Autodesk Inventor part; units mm, degrees
ref_plane "YZ Plane" through (0, 0, 0) normal (1, 0, 0) x (0, 1, 0)
ref_plane "XZ Plane" through (0, 0, 0) normal (0, 1, 0) x (-1, 0, 0)
ref_plane "XY Plane" through (0, 0, 0) normal (0, 0, 1) x (1, 0, 0)
sketch "Schizzo1" plane through (0, 0, 0) normal (0, 0, 1) x (1, 0, 0)
  line L0 (0, 0) -> (90, 0)
  line L1 (90, 0) -> (90, -122)
  line L2 (90, -122) -> (0, -122)
  line L3 (0, -122) -> (0, 0)
  dimension "d0" = 90
  dimension "d1" = 122
extrude "Estrusione1" add sketch "Schizzo1" along normal blind 2.5
sketch "Schizzo2" plane through (0, 0, 2.5) normal (0, 0, 1) x (1, 0, 0)
  line L0 (90, 0) -> (0, 0)
  line L1 (0, -122) -> (90, -122)
  line L2 (90, 0) -> (87, 0)
  line L3 (87, -6.7) -> (12, -6.7)
  line L4 (12, -6.7) -> (12, -41.7)
  line L5 (12, -41.7) -> (87, -41.7)
  line L6 (87, -41.7) -> (87, -6.7)
  line L7 (0, -122) -> (10, -122)
  line L8 (10, -109) -> (83, -109)
  line L9 (83, -109) -> (83, -74)
  line L10 (83, -74) -> (10, -74)
  line L11 (10, -74) -> (10, -109)
  point P0 (87, -6.7)
  dimension "d6" = 75
  dimension "d7" = 35
  dimension "d10" = 73
  dimension "d11" = 35
extrude "Estrusione2" add sketch "Schizzo2" along normal blind 30
sketch "Schizzo3" plane through (0, 0, 2.5) normal (0, 0, 1) x (1, 0, 0)
  line L0 (90, -122) -> (90, 0)
  line L1 (90, 0) -> (0, 0)
  line L2 (90, 0) -> (90, -6)
  line L3 (90, 0) -> (86.5, 0)
  circle A0 centre (86.5, -3.5) radius 2.5
  circle A1 centre (5, -3.5) radius 2.5
  circle A2 centre (5, -103) radius 2.5
  circle A3 centre (86.5, -103) radius 2.5
extrude "Estrusione3" cut sketch "Schizzo3" against normal up to surface (2.5 mm away)
properties part number "PCB" material "Plastica ABS"
Read the model definition and answer for the solid it produces. Units are mm, in the model's axes. A direction names the side the tool comes from. Give positions to 0.01 mm unless a question says otherwise; leave off trailing zeros. Write each loop counter-clockwise with the first axis right and the second up, starting at its lowest first coordinate (ties: lowest second). Pieces come first, ordered by that corner, then holes. Notation, with made-up numbers: (6.25, 47.5) - (58.25, 47.5) arc R17 ccw to (58.25, 51.5) - close; hole circle Ø10 at (13, 67). An arc over 180 degrees is marked (long way). Write item = value, one per line. Start each with the question number.
Item 1: Find section D-D (y = -96). Give the vertices of the cut face in (x, z).
Item 2: Find section B-B (y = -3.5). Give the vertices of the cut face in (x, z), then the cut area to 3 significant figures.
Item 3: A tool of negligible diameter and unlimited length cuts with its end or side. For faces 1 (the flat face through (87, -24, 17)), 2 (the flat face through (12, -24, 17)), 3 (the flat face through (46, -109, 17)), from which of +Z, -Z, +X, -X, +Y, -Y can it reach the whole face along a straight path? Write none if from no direction.
Item 4: Find the intervals of material crossed by probe 1 along Y at (x, z) = (32.5, 12); probe 2 along Y at (x, z) = (11, 28.5); probe 3 along Z at (x, y) = (7.5, -84.5), in increasing order. Write a range as [from, to].
Item 5: Find section A-A (z = 21). Give the vertices of the cut face in (x, y).
Item 6: Find section C-C (x = 5). Give the vertices of the cut face in (y, z).
Item 7: Each of these flat-tipped pins is pushed along its axis until it touches: P1, Ø8, axis at y = -25, z = 23, coming from the -X side; P2, Ø10, axis at x = 62, y = -65.5, coming from the +Z side; P3, Ø10, axis at y = -106.5, z = 11.5, coming from the -X side. Where does it stop, or does it pass through?
Item 8: The mould has two halves that part along Y. Classify faces 4 (the flat face through (47, -74, 17)), 5 (the cylindrical face through (84, -3.4, 1.3)), 6 (the flat face through (50, -6.7, 17)), 7 (the flat face through (83, -92, 17)): +Y half, -Y half, draft (parallel to the pull), parting line (faces both ways), or undercut.
Response:
q1.outline = (0, 0) - (90, 0) - (90, 2.5) - (83, 2.5) - (83, 32.5) - (10, 32.5) - (10, 2.5) - (0, 2.5) - close
q2.outline = (0, 0) - (2.5, 0) - (2.5, 2.5) - (0, 2.5) - close; (7.5, 0) - (84, 0) - (84, 2.5) - (7.5, 2.5) - close; (89, 0) - (90, 0) - (90, 2.5) - (89, 2.5) - close
q2.area = 200 mm²
q3.face_1 = +Z, +X, +Y, -Y
q3.face_2 = +Z, -X, +Y
q3.face_3 = +Z, +X, -X, -Y
q4.probe_1 = [-109, -74], [-41.7, -6.7]
q4.probe_2 = [-109, -74]
q4.probe_3 = [0, 2.5]
q5.outline = (10, -109) - (83, -109) - (83, -74) - (10, -74) - close; (12, -41.7) - (87, -41.7) - (87, -6.7) - (12, -6.7) - close
q6.outline = (-122, 0) - (-105.5, 0) - (-105.5, 2.5) - (-122, 2.5) - close; (-100.5, 0) - (-6, 0) - (-6, 2.5) - (-100.5, 2.5) - close; (-1, 0) - (0, 0) - (0, 2.5) - (-1, 2.5) - close
q7.P1 = 12
q7.P2 = 2.5
q7.P3 = 10
q8.face_4 = undercut
q8.face_5 = undercut
q8.face_6 = +Y half
q8.face_7 = draft
